```python
from build123d import *

# Parameters (mm, degrees)
F2_R     = 3.96875
F3_DEPTH = 3.175
F4_R     = 3.96875
F5_DEPTH = 12.701


with BuildPart() as f1:
    # F0 (on Front) → F1 (revolve)
    with BuildSketch(Plane.XZ):
        with BuildLine():
            Line((-6.218406, 19.05), (-6.218406, 0))
            Line((-6.218406, 0), (6.481594, 0))
            Line((6.481594, 0), (6.481594, 19.05))
            Line((6.481594, 19.05), (3.175, 19.05))
            ThreePointArc((3.175, 19.05), (0, 15.875), (-3.175, 19.05))
            Line((-3.175, 19.05), (-6.218406, 19.05))
        make_face()
    revolve(axis=Axis((0.131594, 0, 0), (1, 0, 0)))

    # F2 (on face) → F3 (cut)
    with BuildSketch(Plane.YZ.offset(6.481594)):
        with BuildLine():
            ThreePointArc((6.35, 17.960512), (0, 19.05), (-6.35, 17.960512))
            Line((-6.35, 17.960512), (-6.35, -17.960512))
            ThreePointArc((-6.35, -17.960512), (0, -19.05), (6.35, -17.960512))
            Line((6.35, -17.960512), (6.35, 17.960512))
        make_face()
        Circle(F2_R, mode=Mode.SUBTRACT)
    extrude(amount=-F3_DEPTH, mode=Mode.SUBTRACT)

    # F4 (on face) → F5 (cut, through all)
    with BuildSketch(Plane(origin=(-6.218406, 0, 0), x_dir=(0, -1, 0), z_dir=(-1, 0, 0))):
        Circle(F4_R)
    extrude(amount=-F5_DEPTH, mode=Mode.SUBTRACT)


solid = f1.part
```
Design review of the part built by this model. Coordinates are the model's own, in mm. A direction names the side the tool comes from. Round coordinates to 2 decimals unless told otherwise and drop trailing zeros. Write each loop counter-clockwise with the first axis right and the second up, starting at its lowest first coordinate (ties: lowest second). Pieces come first, ordered by that corner, then holes.
Item 1: We need section B-B on z = 0. Write out the cut boundary in (x, y) (3 decimals).
Item 2: Clearance check with flat-ended pins moving along their axes: pin 1 Ø1.6 at (x, z) = (5, 7) entering from +Y; pin 2 Ø4 at (x, z) = (2, -1.5) entering from -Y; pin 3 Ø1 at (x, y) = (-2, 6) entering from -Z. State where each tip first meets the part, or that it passes through.
Item 3: For probe 1 along Y at (x, z) = (-3.5, 0); probe 2 along X at (y, z) = (-4, 2), list the stretches that pass through material, from the lowest coordinate up.
Item 4: For faces 1 (the flat face through (5, 6.35, 0)), 2 (the flat face through (6.482, -11, 0)), list the 3-axis set-ups (+Z, -Z, +X, -X, +Y, -Y) from which the entire face can be reached by the end or side of a thin tool; tool diameter is ignored.
Item 5: We need section A-A on y = 0. Write out the cut boundary in (x, z) (3 decimals).
Item 6: We need section C-C on x = -4. Write out the cut boundary in (y, z), and give its area (3 significant figures).
Item 7: The part is to be moulded in two halves that separate along Y. For faces 3 (the flat face through (3.307, 0, 5)), 4 (the flat face through (-6.218, -5, 0)), 5 (the cylindrical face through (4.81, 16.9, 8.79)), 6 (the flat face through (5, -6.35, 0)), say which applies: +Y half, -Y half, draft (parallel to the pull), parting line (faces both ways), or undercut.
Item 8: We need section D-D on x = 4.75. Write out the cut boundary in (y, z).
Returned:
1. outline: (-6.218, -19.05) - (-3.175, -19.05) arc R3.175 cw to (3.175, -19.05) - (6.482, -19.05) - (6.482, -6.35) - (3.307, -6.35) - (3.307, -3.969) - (-6.218, -3.969) - close; (-6.218, 3.969) - (3.307, 3.969) - (3.307, 6.35) - (6.482, 6.35) - (6.482, 19.05) - (3.175, 19.05) arc R3.175 cw to (-3.175, 19.05) - (-6.218, 19.05) - close
2. pin 1: stops at y = 18.01
2. pin 2: stops at y = -19.05
2. pin 3: stops at z = -16.03
3. probe 1: y = -19.05 to -3.97, 3.97 to 19.05
3. probe 2: x = -6.22 to 3.31
4. face 1: +Z, -Z, +X
4. face 2: +Z, -Z, +X, +Y, -Y
5. outline: (-6.218, -19.05) - (-3.175, -19.05) arc R3.175 cw to (3.175, -19.05) - (3.307, -19.05) - (3.307, -3.969) - (-6.218, -3.969) - close; (-6.218, 3.969) - (3.307, 3.969) - (3.307, 19.05) - (3.175, 19.05) arc R3.175 cw to (-3.175, 19.05) - (-6.218, 19.05) - close
6. outline: circle Ø38.1 at (0, 0); hole circle Ø7.94 at (0, 0)
6. area: 1,090 mm2
7. face 3: undercut
7. face 4: draft
7. face 5: parting line
7. face 6: undercut
8. outline: (-6.35, -17.96) - (-6.35, 17.96) arc R19.05 ccw to start; (6.35, -17.96) arc R19.05 ccw to (6.35, 17.96) - close
